from build123d import *

# Parameters (mm, degrees)
BOSS_EXTRUDE1_DEPTH = 14
CUT_EXTRUDE1_REACH  = 39.5
SKETCH2_R           = 2.5
CUT_EXTRUDE2_REACH  = 16
SKETCH3_R           = 6


with BuildPart() as part:
    # Sketch1 → Boss-Extrude1 (new body)
    with BuildSketch(Plane.XY):
        Polygon((0, 0), (0, 6), (11, 6), (11, 37.5), (31, 37.5), (31, 6), (42, 6), (42, 0), align=None)
    extrude(amount=-BOSS_EXTRUDE1_DEPTH)

    # Sketch2 → Cut-Extrude1 (cut, up to next)
    with BuildSketch(Plane.XZ, mode=Mode.PRIVATE) as cut_extrude1_sk1:
        with Locations((5, -7)):
            Circle(SKETCH2_R)
    cut_extrude1_tool1 = extrude(cut_extrude1_sk1.sketch, amount=-CUT_EXTRUDE1_REACH, mode=Mode.PRIVATE) & part.part
    add(cut_extrude1_tool1.solids().sort_by_distance((5, 0, -7))[0], mode=Mode.SUBTRACT)
    # Sketch2 → Cut-Extrude1 (cut, up to next)
    with BuildSketch(Plane.XZ, mode=Mode.PRIVATE) as cut_extrude1_sk2:
        with Locations((37, -7)):
            Circle(SKETCH2_R)
    cut_extrude1_tool2 = extrude(cut_extrude1_sk2.sketch, amount=-CUT_EXTRUDE1_REACH, mode=Mode.PRIVATE) & part.part
    add(cut_extrude1_tool2.solids().sort_by_distance((37, 0, -7))[0], mode=Mode.SUBTRACT)

    # Sketch3 → Cut-Extrude2 (cut, up to next)
    with BuildSketch(Plane.XY, mode=Mode.PRIVATE) as cut_extrude2_sk1:
        with Locations((21, 23)):
            Circle(SKETCH3_R)
    cut_extrude2_tool1 = extrude(cut_extrude2_sk1.sketch, amount=-CUT_EXTRUDE2_REACH, mode=Mode.PRIVATE) & part.part
    add(cut_extrude2_tool1.solids().sort_by_distance((21, 23, 0))[0], mode=Mode.SUBTRACT)


solid = part.part
Here's how the part is built. I have some questions about the finished solid (model axes, mm). A direction names the side the tool comes from. Give positions to 0.01 mm unless a question says otherwise; leave off trailing zeros. Loops run counter-clockwise (first coordinate to the right, second up) from the corner with the lowest first, then second, coordinate; pieces in that order, holes last. Notation, with made-up numbers: (80, -28) -> (92, -28) arc R23 cw to (92, 5) -> close; hole circle Ø1 at (16.25, -39.5). An arc over 180 degrees is marked (long way). Answer as a JSON object with one key per item and string values. Group by question number.
Item 1: I need wall thicknesses on L1, parallel to Y at x = 21, z = -5.5; L2, parallel to Z at x = 5, y = 1.9; L3, parallel to Y at x = 3, z = -4.5. Which ranges of each line are inside material? Lowest first, please.
Item 2: Thinking about a two-plate mould opening in X: for faces 3 (the flat face through (11, 22, -7)), 4 (the cylindrical face through (16.24, 19.35, -6.9)), 5 (the flat face through (8, 6, -7)), 6 (the cylindrical face through (39.31, 2.96, -7.96)), which applies, pulls with the +X half, pulls with the -X half, needs draft (parallel to the pull), parting line crosses it, or undercut?
Item 3: Imagine slicing it at D-D on z = -11. Write out the boundary of the cut face in (x, y).
Item 4: Imagine slicing it at B-B on y = 23. Write out the boundary of the cut face in (x, z).
Item 5: Will these pins go through, and if not, where does the flat tip stop? pin 1 (3.5 mm diameter, centred on x = 36.5, z = -4, fed in from +Y); pin 2 (4 mm diameter, centred on y = 18.5, z = -5, fed in from -X); pin 3 (1 mm diameter, centred on x = 32.5, y = 19.5, fed in from +Z); pin 4 (2 mm diameter, centred on y = 24, z = -2, fed in from +X).
Item 6: Imagine slicing it at A-A on z = -7. Write out the boundary of the cut face in (x, y), then the cut area to 3 significant figures.
Item 7: On a 3-axis mill with a long thin cutter (end or side, diameter ignored), from which of +Z, -Z, +X, -X, +Y, -Y can I reach the whole of each face in a straight line? I mean faces 1 (the flat face through (31, 22, -7)), 2 (the flat face through (21, 37.5, -7)). Say none if no direction works.
Item 8: Imagine slicing it at C-C on x = 5. Write out the boundary of the cut face in (y, z), then the cut area to 3 significant figures.
Answer list:
{
 "1": {"L1": "y = 0 to 17, 29 to 37.5", "L2": "z = -14 to -9.5, -4.5 to 0", "L3": "y = 0 to 6"},
 "2": {"face 3": "pulls with the -X half", "face 4": "undercut", "face 5": "needs draft", "face 6": "undercut"},
 "3": {"outline": "(0, 0) -> (42, 0) -> (42, 6) -> (31, 6) -> (31, 37.5) -> (11, 37.5) -> (11, 6) -> (0, 6) -> close; hole circle Ø12 at (21, 23)"},
 "4": {"outline": "(11, -14) -> (15, -14) -> (15, 0) -> (11, 0) -> close; (27, -14) -> (31, -14) -> (31, 0) -> (27, 0) -> close"},
 "5": {"pin 1": "stops at y = 6", "pin 2": "stops at x = 11", "pin 3": "passes through", "pin 4": "stops at x = 31"},
 "6": {"outline": "(0, 0) -> (2.5, 0) -> (2.5, 6) -> (0, 6) -> close; (7.5, 0) -> (34.5, 0) -> (34.5, 6) -> (31, 6) -> (31, 37.5) -> (11, 37.5) -> (11, 6) -> (7.5, 6) -> close; (39.5, 0) -> (42, 0) -> (42, 6) -> (39.5, 6) -> close; hole circle Ø12 at (21, 23)", "area": "709 mm2"},
 "7": {"face 1": "+Z, -Z, +X, +Y", "face 2": "+Z, -Z, +X, -X, +Y"},
 "8": {"outline": "(0, -14) -> (6, -14) -> (6, -9.5) -> (0, -9.5) -> close; (0, -4.5) -> (6, -4.5) -> (6, 0) -> (0, 0) -> close", "area": "54.0 mm2"}
}
